```python
from build123d import *

# Parameters (mm, degrees)
ESQUISSE1_W         = 86
ESQUISSE1_H         = 70
ESQUISSE1_R         = 2
BOSS_EXTRU_1_DEPTH  = 10
SKETCH1_W           = 2
SKETCH1_H           = 70
BOSS_EXTRUDE2_DEPTH = 10


with BuildPart() as part:
    # Esquisse1 → Boss.-Extru.1 (new body)
    with BuildSketch(Plane.XY):
        with Locations((43, -35)):
            Rectangle(ESQUISSE1_W, ESQUISSE1_H)
        with Locations((3, -17.5)):
            Circle(ESQUISSE1_R, mode=Mode.SUBTRACT)
        with Locations((3, -52.5)):
            Circle(ESQUISSE1_R, mode=Mode.SUBTRACT)
        with Locations((36.4, -52.5)):
            Circle(ESQUISSE1_R, mode=Mode.SUBTRACT)
        with Locations((36.4, -17.5)):
            Circle(ESQUISSE1_R, mode=Mode.SUBTRACT)
        with Locations(Location((49.6, -52.5, 0), (0, 0, 180))):
            Circle(ESQUISSE1_R, mode=Mode.SUBTRACT)
        with Locations(Location((83, -52.5, 0), (0, 0, 180))):
            Circle(ESQUISSE1_R, mode=Mode.SUBTRACT)
        with Locations(Location((83, -17.5, 0), (0, 0, 180))):
            Circle(ESQUISSE1_R, mode=Mode.SUBTRACT)
        with Locations(Location((49.6, -17.5, 0), (0, 0, 180))):
            Circle(ESQUISSE1_R, mode=Mode.SUBTRACT)
    extrude(amount=BOSS_EXTRU_1_DEPTH)

    # Sketch1 → Boss-Extrude2 (add)
    with BuildSketch(Plane(origin=(0, 0, 0), x_dir=(-1, 0, 0), z_dir=(0, 0, -1))):
        with Locations((1, -35)):
            Rectangle(SKETCH1_W, SKETCH1_H)
        with Locations((-87, -35)):
            Rectangle(SKETCH1_W, SKETCH1_H)
    extrude(amount=-BOSS_EXTRUDE2_DEPTH)


solid = part.part
```
Could you check a few things on this model? Use its own coordinates, in mm. Give positions to 0.01 mm unless a question says otherwise; leave off trailing zeros. Write each loop counter-clockwise with the first axis right and the second up, starting at its lowest first coordinate (ties: lowest second). Pieces come first, ordered by that corner, then holes. Notation, with made-up numbers: (12.25, 67.5) - (46.25, 67.5) arc R14 ccw to (46.25, 72.5) - close; hole circle Ø8 at (89.25, 45). An arc over 180 degrees is marked (long way). One line per item, written item: value. Start each with the question number.
Item 1: Imagine slicing it at A-A, the plane x = 3. List the corners of the cut face in (y, z) for me, and give its area (3 significant figures).
Item 2: I'm going to push a flat-ended pin straight in: pin 1 (3.5 mm diameter, centred on x = 49.6, y = -52.5, fed in from -Z). Where does the tip first touch, or does it pass through?
Item 3: Imagine slicing it at C-C, the plane z = 8.75. Give the number of separate pieces and of enclosed holes in the cut face, and give its area (3 significant figures).
Item 4: Please list where these lines run through material, in increasing order: line 1 (Y direction, x = 36.4, z = 5); line 2 (Y direction, x = 37, z = 3.25). Write a range as from..to.
Item 5: Imagine slicing it at B-B, the plane y = -17.5. List the corners of the cut face in (x, z) for me, and give its area (3 significant figures).
Item 6: If we mould it in two halves opening along X, with no side actions, what happens to faces 1 (the face through (49.86, -19.483, 4.93)), 2 (the face through (-2, -35, 5)), 3 (the face through (44, -35, 0))? For each: +X half, -X half, draft (parallel to the pull), parting line (faces both ways), or undercut.
Geometry says:
1. outline: (-70, 0) - (-54.5, 0) - (-54.5, 10) - (-70, 10) - close; (-50.5, 0) - (-19.5, 0) - (-19.5, 10) - (-50.5, 10) - close; (-15.5, 0) - (0, 0) - (0, 10) - (-15.5, 10) - close
1. area: 620 mm^2
2. pin 1: through
3. separate pieces: 1
3. enclosed holes: 8
3. area: 6,200 mm^2
4. line 1: -70..-54.5, -50.5..-19.5, -15.5..0
4. line 2: -70..-54.41, -50.59..-19.41, -15.59..0
5. outline: (-2, 0) - (1, 0) - (1, 10) - (-2, 10) - close; (5, 0) - (34.4, 0) - (34.4, 10) - (5, 10) - close; (38.4, 0) - (47.6, 0) - (47.6, 10) - (38.4, 10) - close; (51.6, 0) - (81, 0) - (81, 10) - (51.6, 10) - close; (85, 0) - (88, 0) - (88, 10) - (85, 10) - close
5. area: 740 mm^2
6. face 1: undercut
6. face 2: -X half
6. face 3: draft
